Check sheet for the modelled part. Datum: model origin and axes. Units: mm. Face numbers are marked on the shaded views. A direction names the side the tool comes from. Give positions to 0.01 mm unless a question says otherwise; leave off trailing zeros. Write each loop counter-clockwise with the first axis right and the second up, starting at its lowest first coordinate (ties: lowest second). Pieces come first, ordered by that corner, then holes. Notation, with made-up numbers: (-2, 37) -> (8, 37) arc R23 cw to (8, 62) -> close; hole circle Ø7 at (12.25, 11.25). An arc over 180 degrees is marked (long way). Return JSON: item names as keys, results as strings.
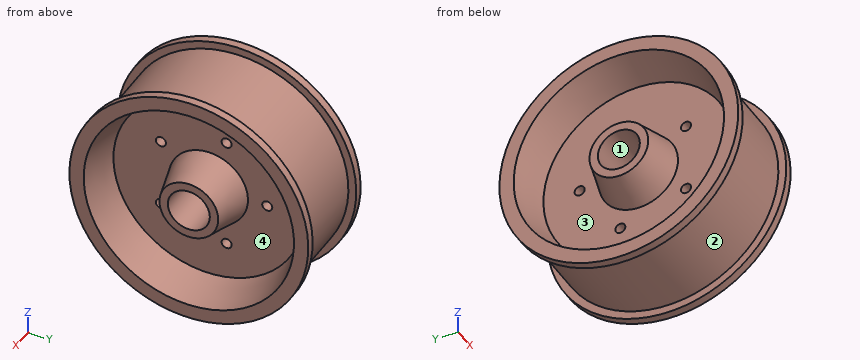
from build123d import *

# Parameters (mm, degrees)
SKETCH2_R          = 3.81
CUT_EXTRUDE1_DEPTH = 137.324658476
CIRPATTERN1_COUNT  = 5


with BuildPart() as part:
    # Sketch1 → Revolve2 (revolve)
    with BuildSketch(Plane.XY, mode=Mode.PRIVATE) as revolve2_sk:
        Polygon((38.1, 90.3224), (31.75, 90.3224), (31.75, 84.380681481), (-31.75, 84.380681481), (-31.75, 90.3224), (-38.1, 90.3224), (-38.1, 79.5274), (-9.525, 71.870751826), (-9.525, 29.881648174), (-38.1, 22.225), (-38.1, 15.875), (38.1, 15.875), (38.1, 22.225), (9.525, 29.881648174), (9.525, 71.870751826), (38.1, 79.5274), align=None)
    revolve(revolve2_sk.sketch.rotate(Axis((-1499.65664488, 0, 0), (1, 0, 0)), 90), axis=Axis((-1499.65664488, 0, 0), (1, 0, 0)))

    # Sketch2 → Cut-Extrude1 (cut, through all)
    with BuildSketch(Plane(origin=(9.525, 0, 0), x_dir=(0, 0, -1), z_dir=(1, 0, 0))):
        with Locations((0, 44.45)):
            Circle(SKETCH2_R)
    cut_extrude1 = extrude(amount=-CUT_EXTRUDE1_DEPTH, mode=Mode.SUBTRACT)

    # CirPattern1: Cut-Extrude1 ×5 about axis
    cirpattern1_axis = Axis((0, 0, 0), (1, 0, 0))
    for i in range(1, CIRPATTERN1_COUNT):
        add(cut_extrude1.rotate(cirpattern1_axis, i * 360 / CIRPATTERN1_COUNT), mode=Mode.SUBTRACT)


solid = part.part
(1) Depth check by flat-ended pin: pin 1 Ø8 at (x, z) = (-7.5, -26) entering from +Y; pin 2 Ø2 at (x, y) = (18, -9) entering from -Z; pin 3 Ø12 at (y, z) = (30.5, -34) entering from -X (3 decimals). Enter the tip coordinate at first touch or a pass-through.
Reply:
{"pin 1": "y = 81.46", "pin 2": "z = -84", "pin 3": "x = -9.525"}
(2) Cross-section at C-C on z = 0. State how many separate pieces and enclosed holes the cut face has, then the cut area to 3 significant figures.
Reply:
{"separate pieces": "3", "enclosed holes": "0", "area": "4,770 mm^2"}
(3) Cross-section at D-D on x = 4. Enter the section's corners in (y, z) (3 decimals), then the cut area to 3 significant figures.
Reply:
{"outline": "circle Ø168.761 at (0, 0); hole circle Ø7.62 at (-35.961, -26.127); hole circle Ø7.62 at (-35.961, 26.127); hole circle Ø31.75 at (0, 0); hole circle Ø7.62 at (13.736, -42.274); hole circle Ø7.62 at (13.736, 42.274); hole circle Ø7.62 at (44.45, 0)", "area": "21,300 mm^2"}
(4) Set-up check for the marked faces 3 and 4: record each of +Z, -Z, +X, -X, +Y, -Y from which the full face is reachable in a straight line by a thin tool's end or side.
Reply:
{"face 3": "-X", "face 4": "+X"}
(5) Thickness scan on L1, parallel to Y at x = 7, z = 0 (3 decimals); L2, parallel to Z at x = 26, y = -21; L3, parallel to Z at x = 14, y = -11. Record the ranges inside material, lowest first.
Reply:
{"L1": "-84.381 to -15.875, 15.875 to 40.64, 48.26 to 84.381", "L2": "-81.73 to -73.34, -14.41 to 14.41, 73.34 to 81.73", "L3": "-83.66 to -72.24, -26.49 to -11.45, 11.45 to 26.49, 72.24 to 83.66"}
(6) Release check for a two-part mould opening along Y. For the marked faces 1 and 2 record: pulls with the +Y half, pulls with the -Y half, needs draft (parallel to the pull), parting line crosses it, or undercut.
Reply:
{"face 1": "undercut", "face 2": "parting line crosses it"}
(7) Cross-section at B-B on x = 16. Enter the section's corners in (y, z) (3 decimals), then the cut area to 3 significant figures.
Reply:
{"outline": "circle Ø168.761 at (0, 0); circle Ø56.293 at (0, 0); hole circle Ø147.211 at (0, 0); hole circle Ø31.75 at (0, 0)", "area": "7,050 mm^2"}
